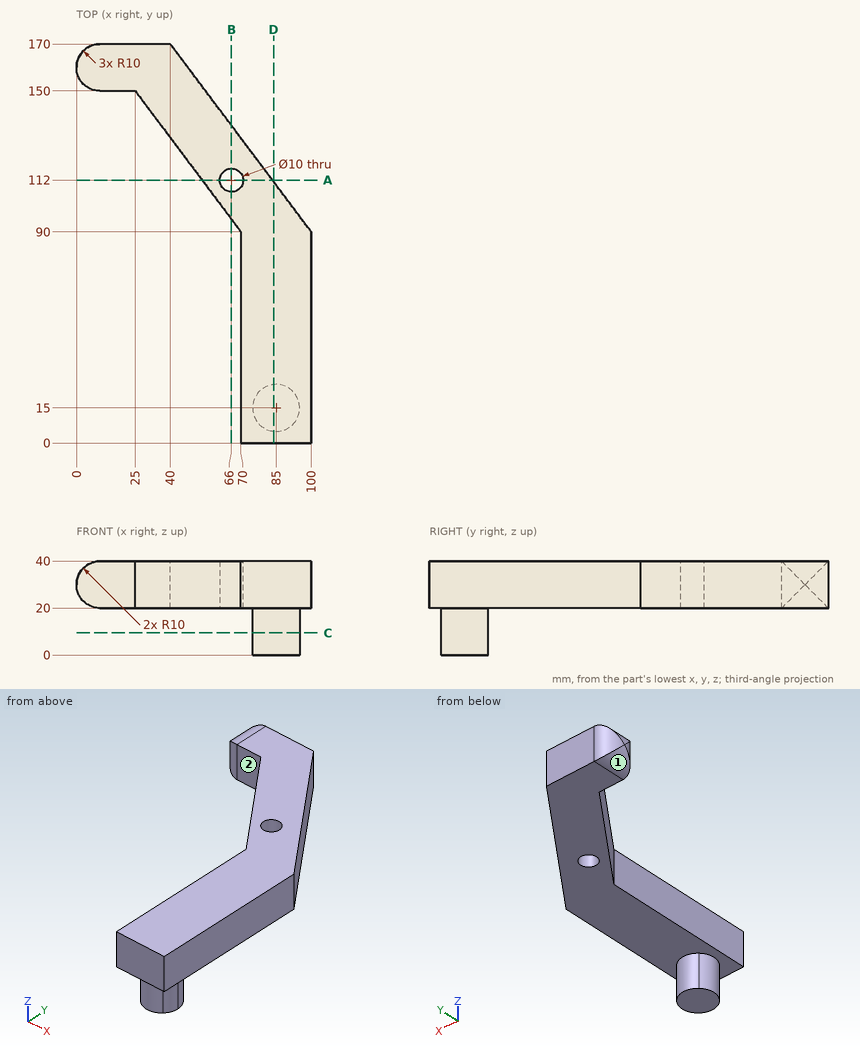
Print and shaded views of the part. All mm, measured from the part's lowest x, y and z. A direction names the side the tool comes from. Coordinates: 2 decimals unless noted, no trailing zeros. Order: outer loops, then holes, each group sorted by start corner. A loop starts at its lowest first (then second) coordinate and runs counter-clockwise, first axis right, second up. Notation, with made-up numbers: (-36, -3.5) -> (-28, -3.5) arc R25 ccw to (-28, 14.5) -> close; hole circle Ø7 at (24.5, 21.5). An arc over 180 degrees is marked (long way). Answer as a JSON object with one key per item and string values. Group by question number.
1) Cut at A-A, the plane y = 112. Write the cut outline in (x, z), then the cut area to 3 significant figures.
2) Flat gauge pins, fed straight in: pin 1 (3 mm diameter, centred on y = 35, z = 26.5, fed in from -X); pin 2 (5 mm diameter, centred on x = 53.5, y = 152.5, fed in from -Z); pin 3 (16.5 mm diameter, centred on x = 18, z = 25.5, fed in from -Y). Where does each tip first touch, or does it go through?
3) Drill centre lines: L1, parallel to X at y = 51, z = 21; L2, parallel to Y at x = 66, z = 25.75; L3, parallel to Y at x = 63, z = 30.5. Where is each one in solid material? Low to high.
4) Cut at B-B, the plane x = 66. Write the cut outline in (y, z).
5) Cut at C-C, the plane z = 9.5. Write the cut outline in (x, y), then the cut area to 3 significant figures.
6) Which spindle directions (+Z, -Z, +X, -X, +Y, -Y) get a long thin tool onto all of the face, cutting with end or side? Do the marked faces 1 and 2. Say none if no direction does.
7) Cut at D-D, the plane x = 84. Write the cut outline in (y, z).
Check values:
{
 "1": {"outline": "(53.5, 20) -> (61, 20) -> (61, 40) -> (53.5, 40) -> close; (71, 20) -> (83.5, 20) -> (83.5, 40) -> (71, 40) -> close", "area": "400 mm²"},
 "2": {"pin 1": "stops at x = 70", "pin 2": "stops at z = 20", "pin 3": "stops at y = 148.33"},
 "3": {"L1": "x = 70 to 100", "L2": "y = 95.33 to 107, 117 to 135.33", "L3": "y = 99.33 to 108, 116 to 139.33"},
 "4": {"outline": "(95.33, 20) -> (107, 20) -> (107, 40) -> (95.33, 40) -> close; (117, 20) -> (135.33, 20) -> (135.33, 40) -> (117, 40) -> close"},
 "5": {"outline": "circle Ø20 at (85, 15)", "area": "314 mm²"},
 "6": {"face 1": "-Z, -X, +Y, -Y", "face 2": "+Z, -Z, -X, -Y"},
 "7": {"outline": "(0, 20) -> (5.05, 20) -> (5.05, 0) -> (24.95, 0) -> (24.95, 20) -> (111.33, 20) -> (111.33, 40) -> (0, 40) -> close"}
}
